```python
from build123d import *

# Parameters (mm, degrees)
F0_R     = 3.3
F0_R_2   = 2.5
F1_DEPTH = 15
F2_R     = 4.25
F3_DEPTH = 7.6
F4_R     = 4.25
F5_DEPTH = 15.8


# Not quite as in the source:
# - a feature names something its author has since deleted; it is built from what else it names


with BuildPart() as f1:
    # F0 (on Right) → F1 (new body)
    with BuildSketch(Plane.YZ):
        with BuildLine():
            ThreePointArc((21.8315579223, 10.717182122), (21.897134346, 10.7177196915), (21.9626931438, 10.7193322557))
            ThreePointArc((21.9626931438, 10.7193322557), (21.9630378123, 10.7252568669), (21.9633808826, 10.731181571))
            ThreePointArc((21.9633808826, 10.731181571), (21.7716697335, 10.7299327404), (21.5799577929, 10.728811993))
            Line((21.5799577929, 10.728811993), (21.8315579223, 10.717182122))
        make_face()
        with BuildLine():
            ThreePointArc((22.1844688263, 10.7327808001), (22.0736743793, 10.7245163933), (21.9626931438, 10.7193322557))
            ThreePointArc((21.9626931438, 10.7193322557), (21.897134346, 10.7177196915), (21.8315579223, 10.717182122))
            ThreePointArc((21.8315579223, 10.717182122), (21.6468606164, 10.7214485341), (21.4625573078, 10.7342386694))
            Line((21.4625573078, 10.7342386694), (-2.0614712889, 11.8216046341))
            ThreePointArc((-2.0614712889, 11.8216046341), (-7.9885695505, -8.9544824829), (11.9792964571, -0.7045966171))
            ThreePointArc((11.9792964571, -0.7045966171), (12.0074816864, -0.4822378377), (12.0652655082, -0.2656763826))
            Line((12.0652655082, -0.2656763826), (12.5823545671, 3.7402298466))
            ThreePointArc((12.5823545671, 3.7402298466), (13.2453067327, 4.9862024463), (14.565897859, 5.4841907695))
            Line((14.565897859, 5.4841907695), (34.746018001, 5.4841907695))
            ThreePointArc((34.746018001, 5.4841907695), (35.4911723527, 5.3401931919), (36.1290262829, 4.9289357615))
            Line((36.1290262829, 4.9289357615), (39.7961525429, 1.4185128035))
            ThreePointArc((39.7961525429, 1.4185128035), (40.4340064731, 1.0072553731), (41.1791608249, 0.8632577956))
            Line((41.1791608249, 0.8632577956), (51.1560065331, 0.8632577956))
            ThreePointArc((51.1560065331, 0.8632577956), (51.3046360431, 0.8687881245), (51.452443583, 0.8853485268))
            Line((51.452443583, 0.8853485268), (68.043755982, 3.3719538424))
            ThreePointArc((68.043755982, 3.3719538424), (68.9480745213, 3.750430082), (69.5639006382, 4.5131846154))
            Line((69.5639006382, 4.5131846154), (71.1927053136, 8.0496168184))
            ThreePointArc((71.1927053136, 8.0496168184), (71.7304115705, 8.7506241115), (72.5176709464, 9.151575379))
            Line((72.5176709464, 9.151575379), (93.0016589096, 14.3460792675))
            ThreePointArc((93.0016589096, 14.3460792675), (93.9531599103, 14.3538506609), (94.800564285, 13.9210454222))
            Line((94.800564285, 13.9210454222), (100.5567479715, 8.9494668086))
            ThreePointArc((100.5567479715, 8.9494668086), (101.3078443235, 8.5419637232), (102.1604743235, 8.4851607509))
            Line((102.1604743235, 8.4851607509), (118.2931486533, 10.9030281733))
            ThreePointArc((118.2931486533, 10.9030281733), (119.516973098, 11.5813971433), (119.9966558679, 12.8958685851))
            ThreePointArc((119.9966558679, 12.8958685851), (119.8113324935, 18.7264110882), (119.3428752162, 24.5410579746))
            ThreePointArc((119.3428752162, 24.5410579746), (118.5020303548, 25.9696085801), (116.872434029, 26.2732411356))
            Line((116.872434029, 26.2732411356), (78.344444671, 16.7187866332))
            ThreePointArc((78.344444671, 16.7187866332), (50.4120849121, 12.3407543123), (22.1844688263, 10.7327808001))
        make_face()
        with BuildLine():
            ThreePointArc((-9.8092514957, -1.9438583008), (-9.6011089256, -1.114801623), (-8.8283263462, -0.7494724707))
            Line((-8.8283263462, -0.7494724707), (-6.2601394612, -0.7494724707))
            ThreePointArc((-6.2601394612, -0.7494724707), (-5.6556353715, -0.9528704337), (-5.2970410826, -1.4803228598))
            ThreePointArc((-5.2970410826, -1.4803228598), (-3.8892204731, -3.8889541154), (-1.4806856428, -5.2969396851))
            ThreePointArc((-1.4806856428, -5.2969396851), (-0.9532704937, -5.6555533383), (-0.7499012145, -6.2600460414))
            Line((-0.7499012145, -6.2600460414), (-0.7499690502, -8.8282543402))
            ThreePointArc((-0.7499690502, -8.8282543402), (-1.1153301427, -9.6010367371), (-1.9444100554, -9.8091421407))
            ThreePointArc((-1.9444100554, -9.8091421407), (-7.0712666783, -7.0708689399), (-9.8092514957, -1.9438583008))
        make_face(mode=Mode.SUBTRACT)
        with BuildLine():
            ThreePointArc((9.8092514957, -1.9438583008), (7.0710678119, -7.0710678119), (1.9438583008, -9.8092514957))
            ThreePointArc((1.9438583008, -9.8092514957), (1.114801623, -9.6011089256), (0.7494724707, -8.8283263462))
            Line((0.7494724707, -8.8283263462), (0.7494724707, -6.2601394612))
            ThreePointArc((0.7494724707, -6.2601394612), (0.9528704337, -5.6556353715), (1.4803228598, -5.2970410826))
            ThreePointArc((1.4803228598, -5.2970410826), (3.8890872965, -3.8890872965), (5.2970410826, -1.4803228598))
            ThreePointArc((5.2970410826, -1.4803228598), (5.6556353715, -0.9528704337), (6.2601394612, -0.7494724707))
            Line((6.2601394612, -0.7494724707), (8.8283263462, -0.7494724707))
            ThreePointArc((8.8283263462, -0.7494724707), (9.6011089256, -1.114801623), (9.8092514957, -1.9438583008))
        make_face(mode=Mode.SUBTRACT)
        Circle(F0_R, mode=Mode.SUBTRACT)
        with BuildLine():
            Line((-6.2601394612, 0.7494724707), (-8.8283263462, 0.7494724707))
            ThreePointArc((-8.8283263462, 0.7494724707), (-9.6011089256, 1.114801623), (-9.8092514957, 1.9438583008))
            ThreePointArc((-9.8092514957, 1.9438583008), (-7.0710799085, 7.0710557152), (-1.9438918628, 9.8092448448))
            ThreePointArc((-1.9438918628, 9.8092448448), (-1.1148229448, 9.6010956435), (-0.7495026768, 8.8282939467))
            Line((-0.7495026768, 8.8282939467), (-0.7495705125, 6.2600856479))
            ThreePointArc((-0.7495705125, 6.2600856479), (-0.9529717251, 5.6556036891), (-1.480405818, 5.2970178982))
            ThreePointArc((-1.480405818, 5.2970178982), (-3.8891177504, 3.8890568424), (-5.2970410826, 1.4803228598))
            ThreePointArc((-5.2970410826, 1.4803228598), (-5.6556353715, 0.9528704337), (-6.2601394612, 0.7494724707))
        make_face(mode=Mode.SUBTRACT)
        with BuildLine():
            Line((0.7494724707, 6.2601394612), (0.7494724707, 8.8283263462))
            ThreePointArc((0.7494724707, 8.8283263462), (1.114801623, 9.6011089256), (1.9438583008, 9.8092514957))
            ThreePointArc((1.9438583008, 9.8092514957), (7.0710678119, 7.0710678119), (9.8092514957, 1.9438583008))
            ThreePointArc((9.8092514957, 1.9438583008), (9.6011089256, 1.114801623), (8.8283263462, 0.7494724707))
            Line((8.8283263462, 0.7494724707), (6.2601394612, 0.7494724707))
            ThreePointArc((6.2601394612, 0.7494724707), (5.6556353715, 0.9528704337), (5.2970410826, 1.4803228598))
            ThreePointArc((5.2970410826, 1.4803228598), (3.8890872965, 3.8890872965), (1.4803228598, 5.2970410826))
            ThreePointArc((1.4803228598, 5.2970410826), (0.9528704337, 5.6556353715), (0.7494724707, 6.2601394612))
        make_face(mode=Mode.SUBTRACT)
        with Locations((50.3031872213, 6.8563437089)):
            Circle(F0_R_2, mode=Mode.SUBTRACT)
        with Locations((111.4225909114, 17.8264938295)):
            Circle(F0_R_2, mode=Mode.SUBTRACT)
        with BuildLine():
            ThreePointArc((21.9633808826, 10.731181571), (21.9630378123, 10.7252568669), (21.9626931438, 10.7193322557))
            ThreePointArc((21.9626931438, 10.7193322557), (22.0736743793, 10.7245163933), (22.1844688263, 10.7327808001))
            ThreePointArc((22.1844688263, 10.7327808001), (22.0739250085, 10.7319598925), (21.9633808826, 10.731181571))
        make_face()
        with BuildLine():
            ThreePointArc((21.4625573078, 10.7342386694), (21.6468606164, 10.7214485341), (21.8315579223, 10.717182122))
            Line((21.8315579223, 10.717182122), (21.5799577929, 10.728811993))
            Line((21.5799577929, 10.728811993), (21.4625573078, 10.7342386694))
        make_face()
    extrude(amount=F1_DEPTH)

    # F2 (on face) → F3 (cut)
    with BuildSketch(Plane(origin=(0, 0, 5.4841907695), x_dir=(1, 0, 0), z_dir=(0, 0, -1))):
        with Locations((7.5, -24.65595793)):
            Circle(F2_R)
    extrude(amount=-F3_DEPTH, mode=Mode.SUBTRACT)

    # F4 (on face) → F5 (cut)
    with BuildSketch(Plane(origin=(0, 2.2011211845, -8.6798933673), x_dir=(1, 0, 0), z_dir=(0, 0.2458080366, -0.9693185282))):
        with Locations((7.5, -84.6746127131)):
            Circle(F4_R)
    extrude(amount=-F5_DEPTH, mode=Mode.SUBTRACT)


solid = f1.part
```
Verification items for the finished model (mm, model axes). A direction names the side the tool comes from. Round coordinates to 2 decimals unless told otherwise and drop trailing zeros. Put each result on its own line as item: value. Start each with the question number.
(1) Section check A-A (x = 9). State how many separate pieces and enclosed holes the cut face has, then the cut area to 3 significant figures.
(2) Draft check along Z on faces 1 (the face through (7, 8, 0.749)), 2 (the face through (7.395, 97.878, 21.563)), 3 (the face through (7.4, 70.37, 6.26)). Enter one of: +Z half, -Z half, draft (parallel to the pull), parting line (faces both ways), or undercut.
(3) Tool access check on faces 4 (the face through (0, 54, 10)), 5 (the face through (4.127, 27.242, 8.136)), 6 (the face through (7, 20, 5.484)), 7 (the face through (7.395, 50.806, 12.383)), 8 (the face through (7.4, -7.01, -7.13)). Record the directions out of +Z, -Z, +X, -X, +Y, -Y that give a thin tool (end or side, any length) a straight path to the whole face; none if there is none.
(4) Depth check by flat-ended pin: pin 1 Ø0.8 at (x, y) = (10.5, -7) entering from +Z; pin 2 Ø2 at (x, z) = (5, -7.5) entering from -Y; pin 3 Ø5 at (x, y) = (4, 45) entering from -Z. Enter the tip coordinate at first touch or a pass-through.
(5) Material ranges on line 1 along Y through (x, z) = (4.75, -6); line 2 along Y through (x, z) = (10.5, -6.5); line 3 along Y through (x, z) = (9.5, 18), recorded low to high.
Completed:
1. separate pieces: 3
1. enclosed holes: 7
1. area: 1,130 mm2
2. face 1: undercut
2. face 2: +Z half
2. face 3: -Z half
3. face 4: +Z, -Z, -X, +Y, -Y
3. face 5: +Z, -Z
3. face 6: -Z, +X, -X
3. face 7: +Z, +X, -X
3. face 8: +X, -X
4. pin 1: stops at z = 10.02
4. pin 2: stops at y = -10.09
4. pin 3: stops at z = 0.86
5. line 1: y = -10.39 to -8, -0.78 to 0.78, 8 to 10.39
5. line 2: y = -10.09 to -7.6, -0.75 to 0.75, 7.6 to 10.09
5. line 3: y = 86.66 to 108.93, 113.92 to 119.85
